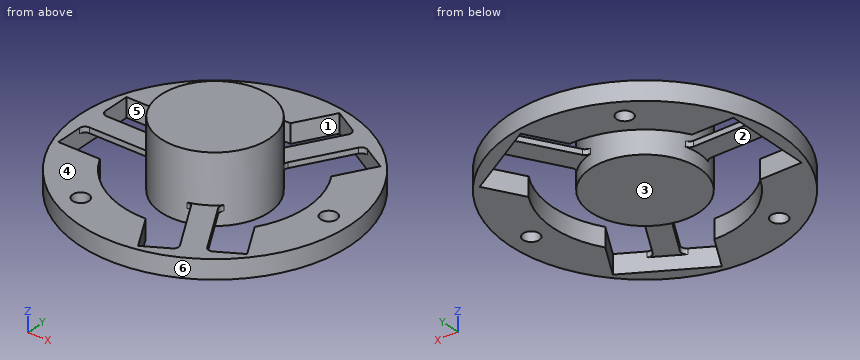
from build123d import *

# Parameters (mm, degrees)
SKETCH1_R                = 10
BOSS_EXTRUDE1_DEPTH      = 9
BOSS_EXTRUDE1_DEPTH_BACK = 3.5
SKETCH1_3_R              = 25
SKETCH1_3_R_2            = 10
BOSS_EXTRUDE2_DEPTH      = 3.5
SKETCH3_R                = 17
CUT_EXTRUDE1_DEPTH       = 3.5
SKETCH8_W                = 9
SKETCH8_H                = 16
CUT_EXTRUDE3_DEPTH       = 4.5
SKETCH10_W               = 12.863801869
SKETCH10_H               = 4
BOSS_EXTRUDE4_DEPTH      = 1
CIRPATTERN2_COUNT        = 3
F_3_0MM_DOWEL_HOLE1_D    = 3
CIRPATTERN3_COUNT        = 3
FILLET1_R                = 1
FILLET2_R                = 1
FILLET3_R                = 1
FILLET4_R                = 1
FILLET5_R                = 1
FILLET6_R                = 1
FILLET7_R                = 1
FILLET8_R                = 1
FILLET9_R                = 1
FILLET10_R               = 1
FILLET11_R               = 1
FILLET12_R               = 1


with BuildPart() as part:
    # Sketch1 → Boss-Extrude1 (new body, two sides)
    with BuildSketch(Plane.XY) as boss_extrude1_sk:
        Circle(SKETCH1_R)
    extrude(amount=BOSS_EXTRUDE1_DEPTH)
    extrude(boss_extrude1_sk.sketch, amount=-BOSS_EXTRUDE1_DEPTH_BACK)



with BuildPart() as body_2:
    # Sketch1<3> → Boss-Extrude2 (new body)
    with BuildSketch(Plane.XY):
        Circle(SKETCH1_3_R)
        Circle(SKETCH1_3_R_2, mode=Mode.SUBTRACT)
    extrude(amount=-BOSS_EXTRUDE2_DEPTH)

    # Sketch3 → Cut-Extrude1 (cut)
    with BuildSketch(Plane.XY):
        Circle(SKETCH3_R)
    extrude(amount=-CUT_EXTRUDE1_DEPTH, mode=Mode.SUBTRACT)

    # Sketch8 → Cut-Extrude3 (cut, through all)
    with BuildSketch(Plane.XY):
        with Locations((-18.16176084, 0)):
            Rectangle(SKETCH8_W, SKETCH8_H)
    cut_extrude3 = extrude(amount=-CUT_EXTRUDE3_DEPTH, mode=Mode.SUBTRACT)


with BuildPart() as part_1:
    add(part.part)

    add(body_2.part)  # Boss-Extrude4 merges body 2
    # Sketch10 → Boss-Extrude4 (add)
    with BuildSketch(Plane.XY):
        with Locations((-16.229859905, 0)):
            Rectangle(SKETCH10_W, SKETCH10_H)
    boss_extrude4 = extrude(amount=-BOSS_EXTRUDE4_DEPTH)

    # CirPattern2: Cut-Extrude3, Boss-Extrude4 ×3 about axis
    cirpattern2_axis = Axis((0, 0, 0), (0, 0, 1))
    for i in range(1, CIRPATTERN2_COUNT):
        add(cut_extrude3.rotate(cirpattern2_axis, i * 360 / CIRPATTERN2_COUNT), mode=Mode.SUBTRACT)
        add(boss_extrude4.rotate(cirpattern2_axis, i * 360 / CIRPATTERN2_COUNT))

    # Ø3.0mm Dowel Hole1 (through all)
    with Locations(Plane.XY):
        with Locations((-10.544029887, 18.161041648)):
            f_3_0mm_dowel_hole1 = Hole(F_3_0MM_DOWEL_HOLE1_D / 2)

    # CirPattern3: Ø3.0mm Dowel Hole1 ×3 about axis
    cirpattern3_axis = Axis((0, 0, 0), (0, 0, 1))
    for i in range(1, CIRPATTERN3_COUNT):
        add(f_3_0mm_dowel_hole1.rotate(cirpattern3_axis, i * 360 / CIRPATTERN3_COUNT), mode=Mode.SUBTRACT)

    # Fillet1
    fillet1_edges = [part_1.edges().sort_by_distance(p)[0] for p in [
        (9.598829613, 20.625660582, -0.5),
    ]]
    fillet(fillet1_edges, radius=FILLET1_R)

    # Fillet2
    fillet2_edges = [part_1.edges().sort_by_distance(p)[0] for p in [
        (13.062931228, 18.625660582, -0.5),
    ]]
    fillet(fillet2_edges, radius=FILLET2_R)

    # Fillet3
    fillet3_edges = [part_1.edges().sort_by_distance(p)[0] for p in [
        (6.631030293, 7.485281374, -0.5),
    ]]
    fillet(fillet3_edges, radius=FILLET3_R)

    # Fillet4
    fillet4_edges = [part_1.edges().sort_by_distance(p)[0] for p in [
        (3.166928678, 9.485281374, -0.5),
    ]]
    fillet(fillet4_edges, radius=FILLET4_R)

    # Fillet5
    fillet5_edges = [part_1.edges().sort_by_distance(p)[0] for p in [
        (-22.66176084, 2, -0.5),
    ]]
    fillet(fillet5_edges, radius=FILLET5_R)

    # Fillet6
    fillet6_edges = [part_1.edges().sort_by_distance(p)[0] for p in [
        (-9.797958971, 2, -0.5),
    ]]
    fillet(fillet6_edges, radius=FILLET6_R)

    # Fillet7
    fillet7_edges = [part_1.edges().sort_by_distance(p)[0] for p in [
        (-22.66176084, -2, -0.5),
    ]]
    fillet(fillet7_edges, radius=FILLET7_R)

    # Fillet8
    fillet8_edges = [part_1.edges().sort_by_distance(p)[0] for p in [
        (-9.797958971, -2, -0.5),
    ]]
    fillet(fillet8_edges, radius=FILLET8_R)

    # Fillet9
    fillet9_edges = [part_1.edges().sort_by_distance(p)[0] for p in [
        (3.166928678, -9.485281374, -0.5),
    ]]
    fillet(fillet9_edges, radius=FILLET9_R)

    # Fillet10
    fillet10_edges = [part_1.edges().sort_by_distance(p)[0] for p in [
        (6.631030293, -7.485281374, -0.5),
    ]]
    fillet(fillet10_edges, radius=FILLET10_R)

    # Fillet11
    fillet11_edges = [part_1.edges().sort_by_distance(p)[0] for p in [
        (9.598829613, -20.625660582, -0.5),
    ]]
    fillet(fillet11_edges, radius=FILLET11_R)

    # Fillet12
    fillet12_edges = [part_1.edges().sort_by_distance(p)[0] for p in [
        (13.062931228, -18.625660582, -0.5),
    ]]
    fillet(fillet12_edges, radius=FILLET12_R)


solid = part_1.part
Source: CAD feature listing. Evaluate the final solid. Frame: model axes, mm. Face numbers are marked on the shaded views. A direction names the side the tool comes from. Give positions to 0.01 mm unless a question says otherwise; leave off trailing zeros. Write each loop counter-clockwise with the first axis right and the second up, starting at its lowest first coordinate (ties: lowest second). Pieces come first, ordered by that corner, then holes. Notation, with made-up numbers: M 74,31.25 L 122,31.25 A20 ccw 122,41.25 Z; hole C 59.25,39 d9. An arc over 180 degrees is marked long. Answer as a JSON object with one key per item and string values.
Q1. Mould query, pull axis Y, two halves, no side actions, for the marked faces 4, 5 and 6. Classes: +Y half, -Y half, draft (parallel to the pull), parting line (faces both ways), or undercut.
Geometry check:
{"face 4": "draft", "face 5": "undercut", "face 6": "parting line"}
Q2. Contact query for flat-ended pins moving along their axis: P1, Ø6, axis at x = 0.5, z = 5.5, coming from the -Y side; P2, Ø2.5, axis at x = -10.54, y = 18.16, coming from the -Z side; P3, Ø5.5, axis at x = 6, y = 17, coming from the -Z side; P4, Ø1, axis at x = -1, z = 7.5, coming from the +Y side. Output: stop coordinate, or through.
Geometry check:
{"P1": "stops at y = -10", "P2": "passes through", "P3": "stops at z = -1", "P4": "stops at y = 9.99"}
Q3. Cut plane A-A, the plane y = 0. Return the cut outline in (x, z), then the cut area to 3 significant figures.
Geometry check:
{"outline": "M -25,-3.5 L -22.66,-3.5 L -22.66,-1 L -10,-1 L -10,-3.5 L 10,-3.5 L 10,9 L -10,9 L -10,0 L -25,0 Z; M 17,-3.5 L 19.5,-3.5 L 19.5,0 L 17,0 Z; M 22.5,-3.5 L 25,-3.5 L 25,0 L 22.5,0 Z", "area": "288 mm^2"}
Q4. Cut plane C-C, the plane z = 2. Return the cut outline in (x, y).
Geometry check:
{"outline": "C 0,0 d20"}
Q5. Cut plane B-B, the plane x = -17. Return the cut outline in (y, z), then the cut area to 3 significant figures.
Geometry check:
{"outline": "M -18.33,-3.5 L -8,-3.5 L -8,0 L -18.33,0 Z; M -2,-1 L 2,-1 L 2,0 L -2,0 Z; M 8,-3.5 L 18.33,-3.5 L 18.33,0 L 8,0 Z", "area": "76.3 mm^2"}
Q6. Ray query, line 1 along X through (y, z) = (8.5, -2.5); line 2 along Z through (x, y) = (9, 17); line 3 along Z through (x, y) = (17, 6). Return the intervals inside material, ascending.
Geometry check:
{"line 1": "x = -23.51 to -14.72, -5.27 to 5.27, 14.72 to 23.51", "line 2": "z = -1 to 0", "line 3": "z = -3.5 to 0"}
Q7. Access query for the marked faces 1, 2 and 3. Directions: +Z, -Z, +X, -X, +Y, -Y. A direction counts if a zero-diameter tool reaches every point of the face in a straight line with its end or side. Return the directions, or none.
Geometry check:
{"face 1": "+Z, -Z", "face 2": "-Z", "face 3": "-Z, +X, -X, +Y, -Y"}
